from build123d import *

# Parameters (mm, degrees)
SKETCH1_R                = 5.75
BOSS_EXTRUDE1_DEPTH      = 14
BOSS_EXTRUDE1_TAPER      = 3
SKETCH2_OUTSIDE_W        = 17.792
SKETCH2_OUTSIDE_H        = 17.792
SKETCH2_OUTSIDE_R        = 3.5
CUT_EXTRUDE1_DEPTH       = 0.4
FILLET2_R                = 1
FILLET3_R                = 1
CUT_EXTRUDE2_DEPTH       = 1
CIRPATTERN1_COUNT        = 6
BOSS_EXTRUDE2_DEPTH      = 1
BOSS_EXTRUDE2_DEPTH_BACK = 1
FILLET4_R                = 1
FILLET5_R                = 0.1
CUT_EXTRUDE3_DEPTH       = 10


with BuildPart() as part:
    # Sketch1 → Boss-Extrude1 (new body)
    with BuildSketch(Plane(origin=(0, 0, 0), x_dir=(1, 0, 0), z_dir=(0, 1, 0))):
        Circle(SKETCH1_R)
    extrude(amount=BOSS_EXTRUDE1_DEPTH, taper=BOSS_EXTRUDE1_TAPER)

    # Sketch2 outside → Cut-Extrude1 (cut)
    with BuildSketch(Plane(origin=(0, 14, 0), x_dir=(1, 0, 0), z_dir=(0, 1, 0))):
        Rectangle(SKETCH2_OUTSIDE_W, SKETCH2_OUTSIDE_H)
        with Locations(Location((0, 0, 0), (0, 0, 270))):
            Circle(SKETCH2_OUTSIDE_R, mode=Mode.SUBTRACT)
    extrude(amount=-CUT_EXTRUDE1_DEPTH, mode=Mode.SUBTRACT)

    # Fillet2
    # the kernel refuses this fillet: 1 mm, written as the material it takes off along each edge
    with BuildSketch(Plane(origin=(0, 14, 0), x_dir=(0, 0, 1), z_dir=(-1, 0, 0))) as fillet2_piece_1:
        with BuildLine():
            CenterArc((2.7, -1), FILLET2_R, 36.869897646, 53.130102354)
            Line((2.7, 0), (2.7, 0.02))
            Line((2.7, 0.02), (3.5, 0.02))
            Line((3.5, 0.02), (3.52, 0))
            ThreePointArc((3.52, 0), (3.52, -0.2), (3.516, -0.388))
            Line((3.516, -0.388), (3.5, -0.4))
        make_face()
    revolve(axis=Axis((0, 14, 0), (0, 1, 0)), mode=Mode.SUBTRACT)

    # Fillet3
    fillet3_edges = [part.edges().sort_by_distance(p)[0] for p in [
        (-5.037254202, 13.6, 0),
    ]]
    fillet(fillet3_edges, radius=FILLET3_R)

    # Sketch3 → Cut-Extrude2 (cut, symmetric)
    with BuildSketch(Plane(origin=(0, 0, 0), x_dir=(0, 0, -1), z_dir=(1, 0, 0))):
        Polygon((-6.905330432, 14.229180533), (-4.800601017, 14.229180533), (-5.581491189, -0.671091575), (-7.885175425, -0.671091575), align=None)
    cut_extrude2 = extrude(amount=CUT_EXTRUDE2_DEPTH, both=True, mode=Mode.SUBTRACT)

    # CirPattern1: Cut-Extrude2 ×6 about axis
    cirpattern1_axis = Axis((0, 0, 0), (0, 1, 0))
    for i in range(1, CIRPATTERN1_COUNT):
        add(cut_extrude2.rotate(cirpattern1_axis, i * 360 / CIRPATTERN1_COUNT), mode=Mode.SUBTRACT)

    # Sketch5 → Boss-Extrude2 (add, two sides: drawn at the far end of the back side and taken through both)
    with BuildSketch(Plane(origin=(0, 0, 0), x_dir=(0, 0, -1), z_dir=(1, 0, 0)).offset(-BOSS_EXTRUDE2_DEPTH_BACK)):
        Polygon((-5.265563969, 0), (-4.679794572, 13.176067739), (-1, 13.176067739), (-1, 14.4), (-5.265563969, 14.4), (-6.009500485, 0), align=None)
    extrude(amount=BOSS_EXTRUDE2_DEPTH + BOSS_EXTRUDE2_DEPTH_BACK)

    # Fillet4
    fillet4_edges = [part.edges().sort_by_distance(p)[0] for p in [
        (0, 14.4, 5.265563969),
    ]]
    fillet(fillet4_edges, radius=FILLET4_R)

    # Fillet5
    fillet5_edges = [part.edges().sort_by_distance(p)[0] for p in [
        (0, 0, 6.009500485),
        (-1, 14.4, 2.657946311),
        (0, 14.4, 1),
        (1, 14.4, 2.657946311),
        (1, 6.725796726, 5.662030639),
        (1, 14.125118422, 5.004516811),
        (-1, 6.725796726, 5.662030639),
        (-1, 14.125118422, 5.004516811),
    ]]
    fillet(fillet5_edges, radius=FILLET5_R)

    # Sketch6 → Cut-Extrude3 (cut)
    with BuildSketch(Plane.XZ):
        with BuildLine():
            Line((-1.5, 2.598076211), (-1.5, -2.598076211))
            ThreePointArc((-1.5, -2.598076211), (3, 0), (-1.5, 2.598076211))
        make_face()
    extrude(amount=-CUT_EXTRUDE3_DEPTH, mode=Mode.SUBTRACT)


solid = part.part
Design review of the part built by this model. Coordinates are the model's own, in mm. A direction names the side the tool comes from. Give positions to 0.01 mm unless a question says otherwise; leave off trailing zeros. Loops run counter-clockwise (first coordinate to the right, second up) from the corner with the lowest first, then second, coordinate; pieces in that order, holes last. Notation, with made-up numbers: M 8.5,42 L 42.5,42 A22 cw 42.5,67 Z; hole C 70,42 d4. An arc over 180 degrees is marked long. Write item = value, one per line.
Q1. For faces 5 (the flat face through (0, 10, 0)), 6 (the conical face through (2.73, 6.415, -4.675)), 7 (the flat face through (0.3, 13.6, -3.7)), list the 3-axis set-ups (+Z, -Z, +X, -X, +Y, -Y) from which the entire face can be reached by the end or side of a thin tool; tool diameter is ignored.
Output values:
face_5 = -Y
face_6 = -Z, +X, +Y
face_7 = +Y
Q2. We need section B-B (z = 0). Give the boundary of the cut face in (x, y), plus the area to 3 significant figures.
Output values:
outline = M -5.75,0 L -1.5,0 L -1.5,10 L 3,10 L 3,0 L 5.75,0 L 5.09,12.65 A1 ccw 4.09,13.6 L 3.5,13.6 A1 ccw 2.7,14 L -2.7,14 A1 ccw -3.5,13.6 L -4.09,13.6 A1 ccw -5.09,12.65 Z
area = 104 mm^2
Q3. We need section A-A (x = 0). Give the boundary of the cut face in (y, z), plus the area to 3 significant figures.
Output values:
outline = M 0,-5.55 L 13.25,-4.85 A1 ccw 13.6,-4.09 L 13.6,-3.5 A1 ccw 14,-2.7 L 14,1 L 14.3,1 A0.1 ccw 14.4,1.1 L 14.4,4.32 A1 ccw 13.45,5.31 L 0.11,6 A0.1 ccw 0,5.9 L 0,3 L 10,3 L 10,-3 L 0,-3 Z
area = 92.4 mm^2
Q4. Insertion check: pin 1 (1.5 mm diameter, centred on y = 7.5, z = -1, fed in from -X); pin 2 (6 mm diameter, centred on y = 6.5, z = 4, fed in from +X); pin 3 (3 mm diameter, centred on x = -1, z = -0.5, fed in from -Y); pin 4 (1.5 mm diameter, centred on x = -2, y = 4.5, fed in from +Z). Each pin has a flat end and moves straight along its axis. Give the tip position at first contact, or say it passes through.
Output values:
pin_1 = -5.37
pin_2 = 5.34
pin_3 = 0
pin_4 = 5.38
Q5. Draft analysis for pull direction Z (two halves, no side actions). For faces 1 (the conical face through (5.414, 6.415, 0.026)), 2 (the cylindrical face through (3, 5, 0)), 3 (the conical face through (2.684, 6.415, 4.702)), 4 (the flat face through (-3, 0, 0)), state which applies: +Z half, -Z half, draft (parallel to the pull), parting line (faces both ways), or undercut.
Output values:
face_1 = parting line
face_2 = undercut
face_3 = +Z half
face_4 = draft
Q6. To check wall thickness, follow line 1 (Y direction, x = 1.25, z = -2.25); line 2 (Z direction, x = 0, y = 1.25); line 3 (X direction, y = 2.5, z = 2). State the ranges of each line that lie inside material, in increasing order. Write a range as [from, to].
Output values:
line_1 = [10, 14]
line_2 = [-5.48, -3], [3, 5.94]
line_3 = [-5.1, -1.5], [2.24, 5.1]
